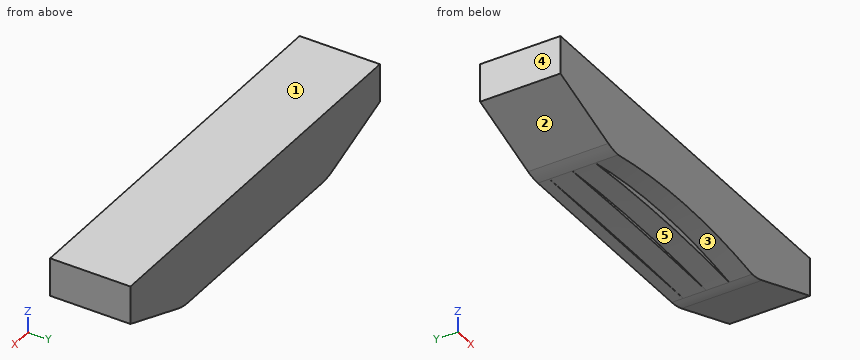
```python
from build123d import *

# Parameters (mm, degrees)
F1_DEPTH = 25.4
F2_R     = 101.6
F4_DEPTH = 50.8
F6_DEPTH = 50.8
F8_DEPTH = 50.8


with BuildPart() as f1:
    # F0 (on Front) → F1 (new body)
    with BuildSketch(Plane.XZ):
        Polygon((-439.8253767191, 78.747405897), (-254, 11.1125), (254, 11.1125), (439.8253767191, 78.747405897), (439.8253767191, 163.5125), (-439.8253767191, 163.5125), align=None)
    extrude(amount=F1_DEPTH)

    # F2
    f2_edges = [f1.edges().sort_by_distance(p)[0] for p in [
        (-254, -12.7, 11.1125),
        (254, -12.7, 11.1125),
    ]]
    fillet(f2_edges, radius=F2_R)

    # F3 (on face) → F4 (join)
    with BuildSketch(Plane.XZ.offset(25.4)):
        with BuildLine():
            ThreePointArc((-236.08517876, 11.1125), (0, 14.2875), (236.08517876, 11.1125))
            ThreePointArc((236.08517876, 11.1125), (253.727833611, 12.656032294), (270.8344253219, 17.2397297282))
            Line((270.8344253219, 17.2397297282), (439.8253767191, 78.747405897))
            Line((439.8253767191, 78.747405897), (439.8253767191, 163.5125))
            Line((439.8253767191, 163.5125), (-439.8253767191, 163.5125))
            Line((-439.8253767191, 163.5125), (-439.8253767191, 78.747405897))
            Line((-439.8253767191, 78.747405897), (-270.8344253219, 17.2397297282))
            ThreePointArc((-270.8344253219, 17.2397297282), (-253.727833611, 12.656032294), (-236.08517876, 11.1125))
        make_face()
    extrude(amount=F4_DEPTH)

    # F5 (on face) → F6 (join)
    with BuildSketch(Plane.XZ.offset(76.2)):
        with BuildLine():
            ThreePointArc((-236.08517876, 11.1125), (0, 20.6375), (236.08517876, 11.1125))
            ThreePointArc((236.08517876, 11.1125), (253.727833611, 12.656032294), (270.8344253219, 17.2397297282))
            Line((270.8344253219, 17.2397297282), (439.8253767191, 78.747405897))
            Line((439.8253767191, 78.747405897), (439.8253767191, 163.5125))
            Line((439.8253767191, 163.5125), (-439.8253767191, 163.5125))
            Line((-439.8253767191, 163.5125), (-439.8253767191, 78.747405897))
            Line((-439.8253767191, 78.747405897), (-270.8344253219, 17.2397297282))
            ThreePointArc((-270.8344253219, 17.2397297282), (-253.727833611, 12.656032294), (-236.08517876, 11.1125))
        make_face()
    extrude(amount=F6_DEPTH)

    # F7 (on face) → F8 (join)
    with BuildSketch(Plane.XZ.offset(127)):
        with BuildLine():
            ThreePointArc((-236.08517876, 11.1125), (0, 33.3375), (236.08517876, 11.1125))
            ThreePointArc((236.08517876, 11.1125), (253.727833611, 12.656032294), (270.8344253219, 17.2397297282))
            Line((270.8344253219, 17.2397297282), (439.8253767191, 78.747405897))
            Line((439.8253767191, 78.747405897), (439.8253767191, 163.5125))
            Line((439.8253767191, 163.5125), (-439.8253767191, 163.5125))
            Line((-439.8253767191, 163.5125), (-439.8253767191, 78.747405897))
            Line((-439.8253767191, 78.747405897), (-270.8344253219, 17.2397297282))
            ThreePointArc((-270.8344253219, 17.2397297282), (-253.727833611, 12.656032294), (-236.08517876, 11.1125))
        make_face()
    extrude(amount=F8_DEPTH)


solid = f1.part
```
Input: part model. Units: mm. Frame: model coordinates. Face numbers are marked on the shaded views. A direction names the side the tool comes from. Round coordinates to 2 decimals unless told otherwise and drop trailing zeros. Write each loop counter-clockwise with the first axis right and the second up, starting at its lowest first coordinate (ties: lowest second). Pieces come first, ordered by that corner, then holes. Notation, with made-up numbers: (26, 61) - (45, 61) arc R36 ccw to (45, 98) - close; hole circle Ø11 at (64.5, -10). An arc over 180 degrees is marked (long way). Write item = value, one per line.
(1) Section query A-A on y = -155.5. Output: boundary loops of the cut face in (x, z).
Geometry check:
outline = (-439.83, 78.75) - (-270.83, 17.24) arc R101.6 ccw to (-236.09, 11.11) arc R1265.02 cw to (236.09, 11.11) arc R101.6 ccw to (270.83, 17.24) - (439.83, 78.75) - (439.83, 163.51) - (-439.83, 163.51) - close
(2) Access query for the marked faces 4 and 5. Directions: +Z, -Z, +X, -X, +Y, -Y. A direction counts if a zero-diameter tool reaches every point of the face in a straight line with its end or side. Return the directions, or none.
Geometry check:
face_4 = +Z, -Z, -X, +Y, -Y
face_5 = -Z, -Y
(3) Pull-direction query (X, two-part tool) for the marked faces 1, 2 and 3; classes: +X half, -X half, draft (parallel to the pull), parting line (faces both ways), or undercut.
Geometry check:
face_1 = draft
face_2 = -X half
face_3 = undercut
(4) Contact query for flat-ended pins moving along their axis: pin 1 Ø3.5 at (x, z) = (62.5, 13) entering from -Y; pin 2 Ø10 at (y, z) = (-50.5, 74) entering from +X; pin 3 Ø10.5 at (x, z) = (-51, 15) entering from -Y. Output: stop coordinate, or through.
Geometry check:
pin_1 = -76.2
pin_2 = 439.83
pin_3 = -127
(5) Section query B-B on x = -27. Output: boundary loops of the cut face in (y, z), then the cut area to 3 significant figures.
Geometry check:
outline = (-177.8, 33.05) - (-127, 33.05) - (-127, 20.51) - (-76.2, 20.51) - (-76.2, 14.25) - (-25.4, 14.25) - (-25.4, 11.11) - (0, 11.11) - (0, 163.51) - (-177.8, 163.51) - close
area = 25,300 mm^2
(6) Material intervals for probe 1 along Z at (x, y) = (5.5, -77.5); probe 2 along Z at (x, y) = (-304, -127), sorted ascending.
Geometry check:
probe_1 = 20.63 to 163.51
probe_2 = 29.31 to 163.51
(7) Section query D-D on z = 56.5. Output: boundary loops of the cut face in (x, y).
Geometry check:
outline = (-378.7, -177.8) - (378.7, -177.8) - (378.7, 0) - (-378.7, 0) - close
(8) Section query C-C on y = -61. Output: boundary loops of the cut face in (x, z), then the cut area to 3 significant figures.
Geometry check:
outline = (-439.83, 78.75) - (-270.83, 17.24) arc R101.6 ccw to (-236.09, 11.11) arc R8778.94 cw to (236.09, 11.11) arc R101.6 ccw to (270.83, 17.24) - (439.83, 78.75) - (439.83, 163.51) - (-439.83, 163.51) - close
area = 120,000 mm^2
